Can you work these out from the model? Positions are in its coordinate system, mm. Face numbers are marked on the shaded views. A direction names the side the tool comes from. Give positions to 0.01 mm unless a question says otherwise; leave off trailing zeros. Write each loop counter-clockwise with the first axis right and the second up, starting at its lowest first coordinate (ties: lowest second). Pieces come first, ordered by that corner, then holes. Notation, with made-up numbers: M 22.25,7 L 33.25,7 A33 ccw 33.25,42 Z; hole C 76.5,-38 d11. An arc over 180 degrees is marked long. Write each question's results on one line, items separated by ' | '.
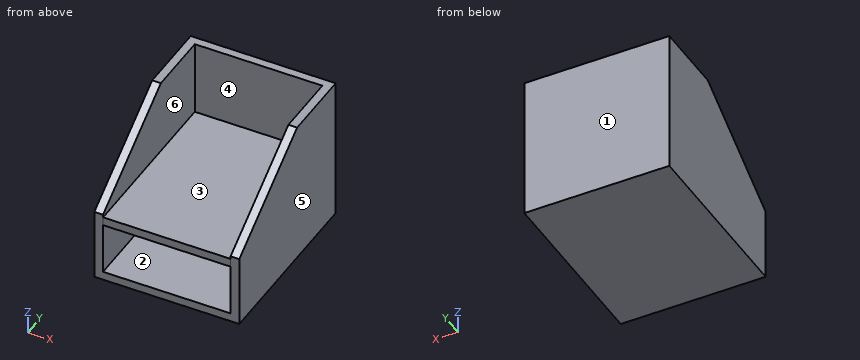
from build123d import *

# Parameters (mm, degrees)
F1_DEPTH = 100
F2_T     = -12
F4_W     = 182.326324
F4_H     = 241.805934
F5_DEPTH = 12


with BuildPart() as f1:
    # F0 (on Right) → F1 (new body, symmetric)
    with BuildSketch(Plane.YZ):
        Polygon((-55.092596, -55.808697), (-55.092596, -155.808697), (194.907404, -155.808697), (194.907404, 44.191303), (94.907404, 44.191303), align=None)
    extrude(amount=F1_DEPTH, both=True)

    # F2
    f2_openings = [f1.faces().sort_by_distance(p)[0] for p in [
        (0, 144.907404, 44.191303),
        (0, 19.907404, -5.808697),
        (0, -55.092596, -105.808697),
    ]]
    offset(amount=F2_T, openings=f2_openings)

    # F4 (on offset) → F5 (join)
    with BuildSketch(Plane.XY.offset(-60)):
        with Locations((0.583131, 65.97941)):
            Rectangle(F4_W, F4_H)
    extrude(amount=-F5_DEPTH)


solid = f1.part
Item 1: I want a section at D-D, the plane y = 5.5. Please give me the cut outline in (x, z), and give its area (3 significant figures).
Geometry says:
outline: M -100,-155.81 L 100,-155.81 L 100,-15.41 L 88,-15.41 L 88,-60 L -88,-60 L -88,-15.41 L -100,-15.41 Z; hole M -88,-143.81 L 88,-143.81 L 88,-72 L -88,-72 Z | area: 7,590 mm2
Item 2: I want a section at B-B, the plane z = -116. Please give me the cut outline in (x, y).
Geometry says:
outline: M -100,-55.09 L -88,-55.09 L -88,182.91 L 88,182.91 L 88,-55.09 L 100,-55.09 L 100,194.91 L -100,194.91 Z
Item 3: I'm going to push flat-ended pins straight in: pin 1 (2 mm diameter, centred on x = 33, y = 7.5, fed in from +Z); pin 2 (1.5 mm diameter, centred on x = -63.5, z = 5, fed in from -Y); pin 3 (6 mm diameter, centred on x = 1.5, z = -68.5, fed in from -Y). Where does each tip first touch, or does it pass through?
Geometry says:
pin 1: stops at z = -60 | pin 2: stops at y = 182.91 | pin 3: stops at y = -54.92
Item 4: For the marked faces 4, 5 and 6, which set-ups out of +Z, -Z, +X, -X, +Y, -Y let a thin tool reach every point of the face, with its end or its side?
Geometry says:
face 4: +Z, -Y | face 5: +Z, -Z, +X, +Y, -Y | face 6: -Y
Item 5: Thinking about a two-plate mould opening in Z: for the marked faces 1, 2 and 3, which applies, +Z half, -Z half, draft (parallel to the pull), parting line (faces both ways), or undercut?
Geometry says:
face 1: draft | face 2: undercut | face 3: +Z half
Item 6: I want a section at C-C, the plane x = 50.5. Please give me the cut outline in (y, z), and give its area (3 significant figures).
Geometry says:
outline: M -55.09,-155.81 L 194.91,-155.81 L 194.91,44.19 L 182.91,44.19 L 182.91,-60 L -54.92,-60 L -54.92,-72 L 182.91,-72 L 182.91,-143.81 L -55.09,-143.81 Z | area: 8,110 mm2
Item 7: If I drill on line 1 (X direction, y = 169.5, z = 10); line 2 (Z direction, x = 61.5, y = 5); line 3 (Y direction, x = -43.5, z = -88), over which ranges is the centre line in solid material (lowest first)? Write a range as from..to.
Geometry says:
line 1: x = -100..-88, 88..100 | line 2: z = -155.81..-143.81, -72..-60 | line 3: y = 182.91..194.91
Item 8: I want a section at A-A, the plane y = 121. Please give me the cut outline in (x, z).
Geometry says:
outline: M -100,-155.81 L 100,-155.81 L 100,44.19 L 88,44.19 L 88,-60 L -88,-60 L -88,44.19 L -100,44.19 Z; hole M -88,-143.81 L 88,-143.81 L 88,-72 L -88,-72 Z
